Autodesk Inventor part; units mm, degrees
ref_plane "YZ Plane" through (0, 0, 0) normal (1, 0, 0) x (0, 1, 0)
ref_plane "XZ Plane" through (0, 0, 0) normal (0, 1, 0) x (-1, 0, 0)
ref_plane "XY Plane" through (0, 0, 0) normal (0, 0, 1) x (1, 0, 0)
sketch "Sketch1" plane through (0, 0, 0) normal (0, 1, 0) x (-1, 0, 0)
  line L0 (-7.5, 10) -> (-1.5, 10)
  line L1 (7.5, 1) -> (7.5, -1)
  line L2 (-1.5, -10) -> (-7.5, -10)
  line L3 (-7.5, -10) -> (-7.5, 10)
  line L4 (-7.5, 10) -> (7.5, -10) construction
  line L5 (7.5, 10) -> (-7.5, -10) construction
  arc A0 (7.5, 1) -> (-1.5, 10) centre (-1.5, 1) ccw
  arc A1 (-1.5, -10) -> (7.5, -1) centre (-1.5, -1) ccw
  point P0 (0, 0)
  dimension "d0" = 15
  dimension "d1" = 20
  dimension "d4" = 9
  dimension "d5" = 9
extrude "Extrusion1" add sketch "Sketch1" along normal blind 25
shell "Shell1" thickness 1 removed faces 1 at (-1.5, 0, 0.3333)
extrude "Extrusion2" add sketch "Sketch1" along normal blind 1
sketch "Sketch2" plane through (1.5, 25, 10) normal (0, 0, 1) x (1, 0, 0)
  line L0 (-9, -25) -> (-9, 0) construction
  line L1 (-9, -25) -> (6, 0) construction
  circle A0 centre (-1.5, -12.5) radius 0.25
  point P0 (-1.5, -25)
  dimension "d9" = 0.5
extrude "Extrusion3" cut sketch "Sketch2" against normal through all
properties part number "actuator_tube_test"
Can you work these out from the model? Positions are in its coordinate system, mm. A direction names the side the tool comes from. Coordinates: 2 decimals unless noted, no trailing zeros. Write each loop counter-clockwise with the first axis right and the second up, starting at its lowest first coordinate (ties: lowest second). Pieces come first, ordered by that corner, then holes. Notation, with made-up numbers: (65, 28.5) - (76, 28.5) arc R16 ccw to (76, 34.5) - close; hole circle Ø6 at (-23, 13.5). An arc over 180 degrees is marked (long way). Return JSON: item names as keys, results as strings.
Q1. If we section it at A-A (z = -0.5): Please give me the cut outline in (x, y), then the cut area to 3 significant figures.
Computed values:
{"outline": "(-7.5, 0) - (7.5, 0) - (7.5, 25) - (-7.5, 25) - close; hole (-6.5, 1) - (6.5, 1) - (6.5, 24) - (-6.5, 24) - close", "area": "76.0 mm2"}
Q2. On a 3-axis mill with a long thin cutter (end or side, diameter ignored), from which of +Z, -Z, +X, -X, +Y, -Y can I reach the whole of each face in a straight line? I mean faces 1 (the cylindrical face through (-4.219, 12.339, -6.594)), 2 (the flat face through (-7.5, 12, 0)). Say none if no direction works.
Computed values:
{"face 1": "none", "face 2": "+Z, -Z, -X, +Y, -Y"}
Q3. If we section it at C-C (y = 10.5): Please give me the cut outline in (x, z), then the cut area to 3 significant figures.
Computed values:
{"outline": "(-7.5, -1) arc R9 ccw to (1.5, -10) - (7.5, -10) - (7.5, 10) - (1.5, 10) arc R9 ccw to (-7.5, 1) - close; hole (-6.5, -1) arc R8 ccw to (1.5, -9) - (6.5, -9) - (6.5, 9) - (1.5, 9) arc R8 ccw to (-6.5, 1) - close", "area": "58.7 mm2"}
Q4. Thinking about a two-plate mould opening in Z: for faces 3 (the cylindrical face through (-4.794, 12.325, 7.434)), 4 (the flat face through (-6.5, 12, 0)), 5 (the cylindrical face through (-4.934, 12.325, -7.294)), which applies, +Z half, -Z half, draft (parallel to the pull), parting line (faces both ways), or undercut?
Computed values:
{"face 3": "+Z half", "face 4": "undercut", "face 5": "-Z half"}
Q5. I'm going to push flat-ended pins straight in: pin 1 Ø3 at (y, z) = (21.5, 6.5) entering from -X; pin 2 Ø4 at (x, y) = (-6, 10.5) entering from -Z. Where does each tip first touch, or does it pass through?
Computed values:
{"pin 1": "stops at x = -6.56", "pin 2": "stops at z = -8.12"}
Q6. Please list where these lines run through material, in increasing order: L1, parallel to Y at x = 0, z = -9.2; L2, parallel to X at y = 13, z = 1.25; L3, parallel to Y at x = -3, z = -2.75. Write a range as from..to.
Computed values:
{"L1": "y = 0..12.25, 12.75..25", "L2": "x = -7.5..-6.5, 6.5..7.5", "L3": "y = 0..1, 24..25"}
Q7. If we section it at B-B (x = 2.5): Please give me the cut outline in (y, z), then the cut area to 3 significant figures.
Computed values:
{"outline": "(0, -10) - (25, -10) - (25, 10) - (0, 10) - close; hole (1, -9) - (24, -9) - (24, 9) - (1, 9) - close", "area": "86.0 mm2"}
